Work out the finished part from the listing and answer in its coordinate system (mm). Face numbers are marked on the shaded views. A direction names the side the tool comes from. Coordinates: 2 decimals unless noted, no trailing zeros. Order: outer loops, then holes, each group sorted by start corner. A loop starts at its lowest first (then second) coordinate and runs counter-clockwise, first axis right, second up. Notation, with made-up numbers: (78, 73) -> (125, 73) arc R32 cw to (125, 107) -> close; hole circle Ø7 at (-2, 82). An arc over 180 degrees is marked (long way). Write item = value, one per line. Start each with the question number.
Q1. The part is cut by section A-A, the plane x = -35. Determine the outline of the cut face in (y, z), plus the area to 3 significant figures.
Q2. The part is cut by section D-D, the plane y = 17.5. Determine the outline of the cut face in (x, z) (3 decimals).
Q3. Which of the six approach directions +Z, -Z, +X, -X, +Y, -Y give full straight-line access (tool end or side, diameter ignored) to the marked faces 1, 2, 3, 4 and 5?
Q4. The part is cut by section B-B, the plane x = -14.5. Determine the outline of the cut face in (y, z).
Q5. For a pull along Z with two mould halves and no side action, classify the marked faces 6, 7 and 8 as +Z half, -Z half, draft (parallel to the pull), parting line (faces both ways), or undercut.
Q6. Flat-ended cylindrical pins translate along their axes: pin 1 (1.8 mm diameter, centred on y = 3, z = -0.5, fed in from -X); pin 2 (10.5 mm diameter, centred on x = 25.5, z = -1.5, fed in from -Y); pin 3 (4 mm diameter, centred on x = -24, z = 10, fed in from -Y). Find the tip coordinate at first contact, or state that the pin passes through.
Q7. Straight lines are drawn through the part: L1, parallel to Z at x = -35, y = -2; L2, parallel to Z at x = -35, y = -10.75; L3, parallel to X at y = 0.5, z = 0. For each, find the intervals that lie inside material, in ascending order. Write a range as from..to.
Q8. The part is cut by section C-C, the plane x = -1. Determine the outline of the cut face in (y, z).
```python
from build123d import *

# Parameters (mm, degrees)
SKETCH1_W                       = 85
SKETCH1_H                       = 30
BOSS_EXTRUDE1_DEPTH             = 20
BOSS_EXTRUDE2_DEPTH             = 85
BOSS_EXTRUDE3_REACH             = 42
BOSS_EXTRUDE3_DIRECTION_2_REACH = 42
SKETCH4_R                       = 3.5
CUT_EXTRUDE1_DEPTH              = 21
SKETCH5_R                       = 9
CUT_EXTRUDE2_DEPTH              = 5
BOSS_EXTRUDE4_DEPTH             = 9
SKETCH6_3_R                     = 9.5
CUT_EXTRUDE3_DEPTH              = 7
SKETCH6_4_R                     = 9.5
SKETCH6_4_R_2                   = 3.5
BOSS_EXTRUDE5_DEPTH             = 6
SKETCH8_R                       = 10
SKETCH8_R_2                     = 9.5
BOSS_EXTRUDE6_DEPTH             = 13
CUT_EXTRUDE4_DEPTH              = 5
CUT_EXTRUDE4_DEPTH_BACK         = 40
SKETCH10_W                      = 34.61835073
SKETCH10_H                      = 46.546399138
CUT_EXTRUDE5_DEPTH              = 6


with BuildPart() as part:
    # Sketch1 → Boss-Extrude1 (new body)
    with BuildSketch(Plane(origin=(0, 0, 0), x_dir=(1, 0, 0), z_dir=(0, 1, 0))):
        Rectangle(SKETCH1_W, SKETCH1_H)
    extrude(amount=BOSS_EXTRUDE1_DEPTH)

    # Sketch2 → Boss-Extrude2 (add)
    with BuildSketch(Plane(origin=(42.5, 0, 0), x_dir=(0, 0, -1), z_dir=(1, 0, 0))):
        Polygon((15, 20), (40, 0), (15, 0), align=None)
        Polygon((-15, 20), (-40, 0), (-15, 0), align=None)
    extrude(amount=-BOSS_EXTRUDE2_DEPTH)

    # Boss-Extrude3: up to this face of the body (flat: up to its plane)
    boss_extrude3_end = Plane(part.part.faces().sort_by_distance((0, 10, -27.5))[0])
    # Sketch3 → Boss-Extrude3 (add, up to the picked face)
    with BuildSketch(Plane.XY, mode=Mode.PRIVATE) as boss_extrude3_sk1:
        Polygon((42.5, 20), (50.5, 0), (42.5, 0), align=None)
    boss_extrude3_tool1 = split(extrude(boss_extrude3_sk1.sketch, amount=-BOSS_EXTRUDE3_REACH, mode=Mode.PRIVATE), bisect_by=boss_extrude3_end, keep=Keep.BOTH, mode=Mode.PRIVATE)
    add(boss_extrude3_tool1.solids().sort_by_distance((45.166667, 6.666667, 0))[0])
    # Sketch3 → Boss-Extrude3 (add, up to the picked face)
    with BuildSketch(Plane.XY, mode=Mode.PRIVATE) as boss_extrude3_sk2:
        Polygon((-42.5, 0), (-42.5, 20), (-50.5, 0), align=None)
    boss_extrude3_tool2 = split(extrude(boss_extrude3_sk2.sketch, amount=-BOSS_EXTRUDE3_REACH, mode=Mode.PRIVATE), bisect_by=boss_extrude3_end, keep=Keep.BOTH, mode=Mode.PRIVATE)
    add(boss_extrude3_tool2.solids().sort_by_distance((-45.166667, 6.666667, 0))[0])

    # Boss-Extrude3 direction 2: up to this face of the body (flat: up to its plane)
    boss_extrude3_direction_2_end = Plane(part.part.faces().sort_by_distance((0, 10, 27.5))[0])
    # Sketch3 → Boss-Extrude3 direction 2 (add, up to the picked face)
    with BuildSketch(Plane.XY, mode=Mode.PRIVATE) as boss_extrude3_direction_2_sk1:
        Polygon((42.5, 20), (50.5, 0), (42.5, 0), align=None)
    boss_extrude3_direction_2_tool1 = split(extrude(boss_extrude3_direction_2_sk1.sketch, amount=BOSS_EXTRUDE3_DIRECTION_2_REACH, mode=Mode.PRIVATE), bisect_by=boss_extrude3_direction_2_end, keep=Keep.BOTH, mode=Mode.PRIVATE)
    add(boss_extrude3_direction_2_tool1.solids().sort_by_distance((45.166667, 6.666667, 0))[0])
    # Sketch3 → Boss-Extrude3 direction 2 (add, up to the picked face)
    with BuildSketch(Plane.XY, mode=Mode.PRIVATE) as boss_extrude3_direction_2_sk2:
        Polygon((-42.5, 0), (-42.5, 20), (-50.5, 0), align=None)
    boss_extrude3_direction_2_tool2 = split(extrude(boss_extrude3_direction_2_sk2.sketch, amount=BOSS_EXTRUDE3_DIRECTION_2_REACH, mode=Mode.PRIVATE), bisect_by=boss_extrude3_direction_2_end, keep=Keep.BOTH, mode=Mode.PRIVATE)
    add(boss_extrude3_direction_2_tool2.solids().sort_by_distance((-45.166667, 6.666667, 0))[0])

    # Sketch4 → Cut-Extrude1 (cut, through all)
    with BuildSketch(Plane(origin=(0, 20, 0), x_dir=(1, 0, 0), z_dir=(0, 1, 0))):
        with Locations((-14.5, 0)):
            Circle(SKETCH4_R)
    extrude(amount=-CUT_EXTRUDE1_DEPTH, mode=Mode.SUBTRACT)

    # Sketch5 → Cut-Extrude2 (cut)
    with BuildSketch(Plane(origin=(0, 20, 0), x_dir=(1, 0, 0), z_dir=(0, 1, 0))):
        with Locations((-14.5, 0)):
            Circle(SKETCH5_R)
    extrude(amount=-CUT_EXTRUDE2_DEPTH, mode=Mode.SUBTRACT)

    # Sketch6 → Boss-Extrude4 (add)
    with BuildSketch(Plane.XZ):
        with BuildLine():
            Line((-7.5, 5), (-32.968954756, 8.36635465))
            ThreePointArc((-32.968954756, 8.36635465), (-50.488194155, -7.60484858), (-31.776786955, -22.161164126))
            Line((-31.776786955, -22.161164126), (-7.5, -17))
            Line((-7.5, -17), (-7.5, 5))
        make_face()
        with BuildLine():
            ThreePointArc((-33.23102511, 6.383599211), (-48.48971749, -7.526803602), (-32.192685412, -20.204884884))
            Line((-32.192685412, -20.204884884), (-9.5, -15.380495475))
            Line((-9.5, -15.380495475), (-9.5, 3.246955109))
            Line((-9.5, 3.246955109), (-33.23102511, 6.383599211))
        make_face(mode=Mode.SUBTRACT)
    extrude(amount=BOSS_EXTRUDE4_DEPTH)

    # Sketch6<3> → Cut-Extrude3 (cut)
    with BuildSketch(Plane.XZ):
        with Locations((-35, -7)):
            Circle(SKETCH6_3_R)
    extrude(amount=-CUT_EXTRUDE3_DEPTH, mode=Mode.SUBTRACT)

    # Sketch6<4> → Boss-Extrude5 (add)
    with BuildSketch(Plane.XZ):
        with BuildLine():
            Line((-9.5, 3.246955109), (-33.23102511, 6.383599211))
            ThreePointArc((-33.23102511, 6.383599211), (-48.48971749, -7.526803602), (-32.192685412, -20.204884884))
            Line((-32.192685412, -20.204884884), (-9.5, -15.380495475))
            Line((-9.5, -15.380495475), (-9.5, 3.246955109))
        make_face()
        with Locations((-35, -7)):
            Circle(SKETCH6_4_R, mode=Mode.SUBTRACT)
        with Locations((-14.5, 0)):
            Circle(SKETCH6_4_R_2, mode=Mode.SUBTRACT)
    extrude(amount=BOSS_EXTRUDE5_DEPTH)

    # Sketch8 → Boss-Extrude6 (add)
    with BuildSketch(Plane.XZ.offset(6)):
        with Locations((-35, -7)):
            Circle(SKETCH8_R)
        with Locations((-35, -7)):
            Circle(SKETCH8_R_2, mode=Mode.SUBTRACT)
    extrude(amount=BOSS_EXTRUDE6_DEPTH)

    # Sketch9 → Cut-Extrude4 (cut, two sides)
    with BuildSketch(Plane(origin=(0, 0, 0), x_dir=(0, 0, -1), z_dir=(1, 0, 0))) as cut_extrude4_sk:
        Polygon((33.848828411, 3), (-33.848828411, 3), (-18.848828411, 15), (18.848828411, 15), align=None)
    extrude(amount=CUT_EXTRUDE4_DEPTH, mode=Mode.SUBTRACT)
    extrude(cut_extrude4_sk.sketch, amount=-CUT_EXTRUDE4_DEPTH_BACK, mode=Mode.SUBTRACT)

    # Sketch10 → Cut-Extrude5 (cut)
    with BuildSketch(Plane(origin=(0, 0, 0), x_dir=(-1, 0, 0), z_dir=(0, -1, 0))):
        with Locations((-25.663362502, 2.40647956)):
            Rectangle(SKETCH10_W, SKETCH10_H)
    extrude(amount=-CUT_EXTRUDE5_DEPTH, mode=Mode.SUBTRACT)


solid = part.part
```
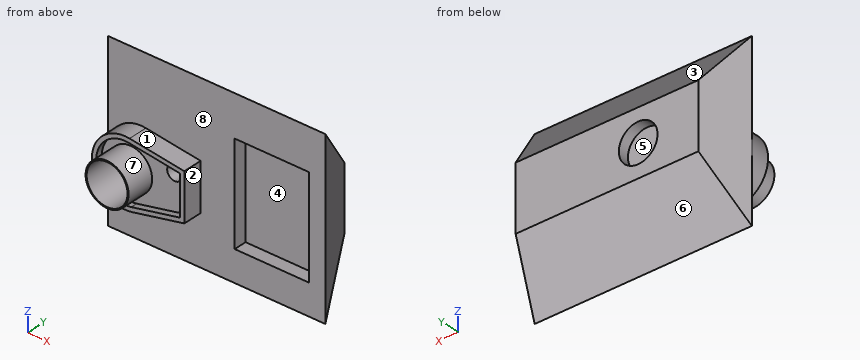
Model answer:
q1.outline = (-19, -17) -> (-6, -17) -> (-6, -20.5) -> (-9, -20.5) -> (-9, -22.5) -> (0, -22.5) -> (0, -40) -> (20, -15) -> (20, 15) -> (0, 40) -> (0, 8.5) -> (-9, 8.5) -> (-9, 6.5) -> (-6, 6.5) -> (-6, 3) -> (-19, 3) -> (-19, 2.5) -> (3, 2.5) -> (3, 33.85) -> (15, 18.85) -> (15, -18.85) -> (3, -33.85) -> (3, -16.5) -> (-19, -16.5) -> close
q1.area = 508 mm2
q2.outline = (-43.5, -18.125) -> (43.5, -18.125) -> (43.5, 18.125) -> (-43.5, 18.125) -> close; hole circle Ø18 at (-14.5, 0)
q3.face_1 = +Z, +X, -Y
q3.face_2 = +Z, -Z, +X, -Y
q3.face_3 = +Z, +X, -X, +Y
q3.face_4 = -Y
q3.face_5 = none
q4.outline = (-9, -18.49) -> (0, -18.49) -> (0, -40) -> (20, -15) -> (20, -9) -> (15, -9) -> (15, -18.85) -> (3, -33.85) -> (3, -3.5) -> (-6, -3.5) -> (-6, -16.44) -> (-9, -16.44) -> close; (-9, 3.91) -> (-6, 3.91) -> (-6, 3.5) -> (3, 3.5) -> (3, 33.85) -> (15, 18.85) -> (15, 9) -> (20, 9) -> (20, 15) -> (0, 40) -> (0, 5.93) -> (-9, 5.93) -> close
q5.face_6 = -Z half
q5.face_7 = undercut
q5.face_8 = draft
q6.pin_1 = -49.66
q6.pin_2 = 6
q6.pin_3 = 0
q7.L1 = -22.5..-16.5, 2.5..8.5
q7.L2 = -17..-16.5, 2.5..3
q7.L3 = -50.3..-41.42, -28.58..-18, -11..8.35, 42.97..50.3
q8.outline = (0, -40) -> (20, -15) -> (20, 15) -> (0, 40) -> close; hole (3, -33.85) -> (15, -18.85) -> (15, 18.85) -> (3, 33.85) -> close
